Model file for the job. Use its own axes, mm. Face numbers are marked on the shaded views. A direction names the side the tool comes from. Coordinates: 2 decimals unless noted, no trailing zeros. Write each loop counter-clockwise with the first axis right and the second up, starting at its lowest first coordinate (ties: lowest second). Pieces come first, ordered by that corner, then holes. Notation, with made-up numbers: M 69,-4 L 89,-4 A14 ccw 89,6 Z; hole C 57,56.5 d9. An arc over 180 degrees is marked long. One line per question, with ' | ' between items. Start each with the question number.
(1) Cut at C-C (y = -0.25). Write the cut outline in (x, z).
(2) Cut at D-D (z = 5). Write the cut outline in (x, y), plus the area to 3 significant figures.
(3) Wall check: probe 1 along Z at (x, y) = (3.5, 3.25); probe 2 along X at (y, z) = (5.75, -2.5); probe 3 along Z at (x, y) = (0.5, -1.5). Give the ranges that are in metal, low to high.
(4) Flat gauge pins, fed straight in: pin 1 Ø6 at (y, z) = (0, -1) entering from +X; pin 2 Ø0.9 at (y, z) = (0.5, -3) entering from -X; pin 3 Ø3 at (x, y) = (-2, -0.5) entering from -Z; pin 4 Ø5 at (x, y) = (-2.5, -4) entering from -Z. Where does each tip first touch, or does it go through?
(5) Cut at A-A (z = 0.75). Write the cut outline in (x, y).
(6) Tool access for the marked faces 4, 5, 6, 7 and 8: list every direction of +Z, -Z, +X, -X, +Y, -Y with a clear straight run to the whole face (end or side of a thin tool).
(7) Cut at B-B (x = -3). Write the cut outline in (y, z), plus the area to 3 significant figures.
(8) Two-plate mould, pull along Z, no slides. Class the marked faces 1, 2 and 3: +Z half, -Z half, draft (parallel to the pull), parting line (faces both ways), or undercut.
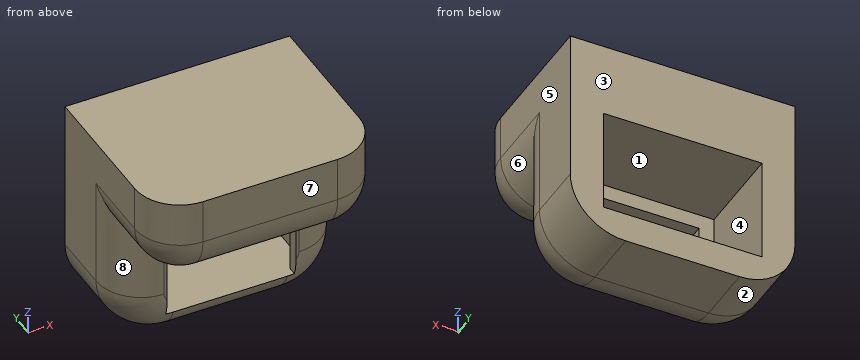
from build123d import *

# Parameters (mm, degrees)
SKETCH1_W           = 15
SKETCH1_H           = 14
BOSS_EXTRUDE1_DEPTH = 7
FILLET1_R           = 3.7
SKETCH2_W           = 10.6
SKETCH2_H           = 7
CUT_EXTRUDE1_DEPTH  = 6.2
SKETCH3_W           = 8.6
SKETCH3_H           = 6
CUT_EXTRUDE2_DEPTH  = 12.987076374
SKETCH4_W           = 15
SKETCH4_H           = 6
BOSS_EXTRUDE2_DEPTH = 5
FILLET8_R           = 3
FILLET9_R           = 3
FILLET10_R          = 3


with BuildPart() as part:
    # Sketch1 → Boss-Extrude1 (new body)
    with BuildSketch(Plane(origin=(0, 0, 0), x_dir=(1, 0, 0), z_dir=(0, 1, 0))):
        Rectangle(SKETCH1_W, SKETCH1_H)
    extrude(amount=BOSS_EXTRUDE1_DEPTH)

    # Fillet1
    fillet1_edges = [part.edges().sort_by_distance(p)[0] for p in [
        (-7.5, 3.5, -7),
        (7.5, 3.5, -7),
    ]]
    fillet(fillet1_edges, radius=FILLET1_R)

    # Sketch2 → Cut-Extrude1 (cut)
    with BuildSketch(Plane(origin=(0, 7, 0), x_dir=(1, 0, 0), z_dir=(0, 1, 0))):
        with Locations((0, 1.5)):
            Rectangle(SKETCH2_W, SKETCH2_H)
    extrude(amount=-CUT_EXTRUDE1_DEPTH, mode=Mode.SUBTRACT)

    # Sketch3 → Cut-Extrude2 (cut, through all)
    with BuildSketch(Plane(origin=(0, 0.8, 0), x_dir=(1, 0, 0), z_dir=(0, 1, 0))):
        with Locations((0, 2)):
            Rectangle(SKETCH3_W, SKETCH3_H)
    extrude(amount=-CUT_EXTRUDE2_DEPTH, mode=Mode.SUBTRACT)

    # Sketch4 → Boss-Extrude2 (add)
    with BuildSketch(Plane.XZ):
        with Locations((0, 4)):
            Rectangle(SKETCH4_W, SKETCH4_H)
    extrude(amount=BOSS_EXTRUDE2_DEPTH)

    # Fillet8
    fillet8_edges = [part.edges().sort_by_distance(p)[0] for p in [
        (-7.5, -5, 4),
        (7.5, -5, 4),
    ]]
    fillet(fillet8_edges, radius=FILLET8_R)

    # Fillet9
    # the kernel refuses this fillet: 3 mm, written as the material it takes off along each edge
    with BuildSketch(Plane(origin=(-3.8, 0, -3.3), x_dir=(0, 0, -1), z_dir=(1, 0, 0))) as fillet9_piece_1:
        with BuildLine():
            CenterArc((3.7 - FILLET9_R, FILLET9_R), FILLET9_R, 270, 90)
            Line((3.7, FILLET9_R), (3.7, 0))
            Line((3.7, 0), (3.7 - FILLET9_R, 0))
        make_face()
    revolve(axis=Axis((-3.8, 0, -3.3), (0, 1, 0)), revolution_arc=90, mode=Mode.SUBTRACT)
    with BuildSketch(Plane(origin=(3.8, 0, -3.3), x_dir=(0, 0, -1), z_dir=(-1, 0, 0))) as fillet9_piece_2:
        with BuildLine():
            CenterArc((3.7 - FILLET9_R, -FILLET9_R), FILLET9_R, 0, 90)
            Line((3.7, -FILLET9_R), (3.7, 0))
            Line((3.7, 0), (3.7 - FILLET9_R, 0))
        make_face()
    revolve(axis=Axis((3.8, 0, -3.3), (0, -1, 0)), revolution_arc=90, mode=Mode.SUBTRACT)
    with BuildSketch(Plane(origin=(-7.5, 0, 1), x_dir=(0, 1, 0), z_dir=(0, 0, -1))) as fillet9_piece_3:
        with BuildLine():
            CenterArc((FILLET9_R, FILLET9_R), FILLET9_R, 180, 90)
            Line((0, FILLET9_R), (0, 0))
            Line((0, 0), (FILLET9_R, 0))
        make_face()
    extrude(amount=4.3, mode=Mode.SUBTRACT)
    with BuildSketch(Plane(origin=(7.5, 0, -3.3), x_dir=(-1, 0, 0), z_dir=(0, 0, 1))) as fillet9_piece_4:
        with BuildLine():
            CenterArc((FILLET9_R, -FILLET9_R), FILLET9_R, 90, 90)
            Line((0, -FILLET9_R), (0, 0))
            Line((0, 0), (FILLET9_R, 0))
        make_face()
    extrude(amount=4.3, mode=Mode.SUBTRACT)
    with BuildSketch(Plane(origin=(-3.8, 0, -7), x_dir=(0, 0, 1), z_dir=(1, 0, 0))) as fillet9_piece_5:
        with BuildLine():
            CenterArc((FILLET9_R, -FILLET9_R), FILLET9_R, 90, 90)
            Line((0, -FILLET9_R), (0, 0))
            Line((0, 0), (FILLET9_R, 0))
        make_face()
    extrude(amount=7.6, mode=Mode.SUBTRACT)

    # Fillet10
    fillet10_edges = [part.edges().sort_by_distance(p)[0] for p in [
        (0, -5, 1),
        (7.5, 0.5, 1),
        (-7.5, 0.5, 1),
        (6.621320344, -4.121320344, 1),
        (-6.621320344, -4.121320344, 1),
    ]]
    fillet(fillet10_edges, radius=FILLET10_R)


solid = part.part
Filled in:
1) outline: M -7.5,4 A3 ccw -4.5,1 L 4.5,1 A3 ccw 7.5,4 L 7.5,7 L -7.5,7 Z
2) outline: M -7.5,-2 A3 ccw -4.5,-5 L 4.5,-5 A3 ccw 7.5,-2 L 7.5,7 L -7.5,7 Z | area: 176 mm²
3) probe 1: -7 to -5, 2 to 7 | probe 2: -7.5 to -5.3, 5.3 to 7.5 | probe 3: 1 to 7
4) pin 1: x = 7.5 | pin 2: x = -6.69 | pin 3: z = -6.24 | pin 4: z = 1
5) outline: M -7.5,3 A3 ccw -4.5,0 L -4.3,0 L -4.3,0.8 L -5.3,0.8 L -5.3,7 L -7.5,7 Z; M 4.3,0 L 4.5,0 A3 ccw 7.5,3 L 7.5,7 L 5.3,7 L 5.3,0.8 L 4.3,0.8 Z
6) face 4: +Y | face 5: +Z, -Z, +X, +Y, -Y | face 6: -Z, +X, -Y | face 7: +Z, -Z, +X, -X, -Y | face 8: -Z, -X, -Y
7) outline: M -5,4 A3 ccw -2,1 L 0.8,1 L 0.8,2 L 7,2 L 7,7 L -5,7 Z; M 0.17,-5 A3 ccw 3,-7 L 7,-7 L 7,-5 Z | area: 76.0 mm²
8) face 1: undercut | face 2: -Z half | face 3: draft
